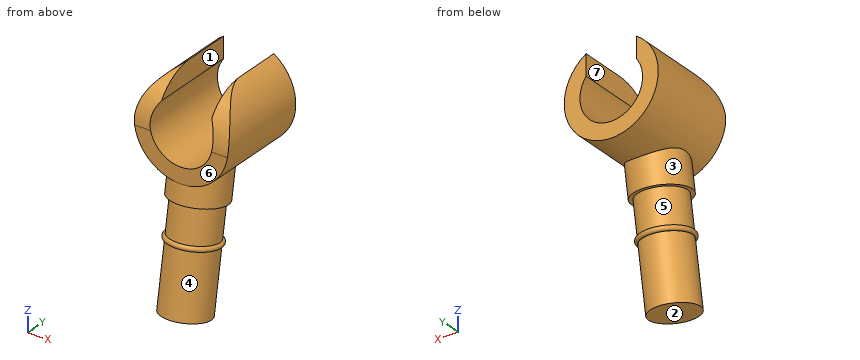
from build123d import *

# Parameters (mm, degrees)
SKETCH2_R                = 2.38125
SKETCH2_R_2              = 1.5875000000000001
BOSS_EXTRUDE1_DEPTH      = 4.7625
SKETCH3_W                = 2.54
SKETCH3_H                = 2.54
CUT_EXTRUDE1_DEPTH       = 6.832847450002443
CUT_EXTRUDE2_DEPTH       = 7.456267061932925
CUT_EXTRUDE2_DEPTH_BACK  = 7.456267061932925
BOSS_EXTRUDE2_REACH      = 13.721
BOSS_EXTRUDE2_END_RADIUS = 2.38125
SKETCH6_R                = 1.1906250000000003
BOSS_EXTRUDE3_REACH      = 19.432
BOSS_EXTRUDE3_END_RADIUS = 2.38125
BOSS_EXTRUDE3_START      = -5.159375
SKETCH7_R                = 1.3881469237206399
SKETCH8_R                = 0.1270000000001564


with BuildPart() as part:
    # Sketch2 → Boss-Extrude1 (new body)
    with BuildSketch(Plane(origin=(0, 0, 0), x_dir=(1, 0, 0), z_dir=(0, 1, 0))):
        with Locations(Location((0, 0, 0), (0, 0, 90))):
            Circle(SKETCH2_R)
        with Locations(Location((0, 0, 0), (0, 0, 90))):
            Circle(SKETCH2_R_2, mode=Mode.SUBTRACT)
    extrude(amount=BOSS_EXTRUDE1_DEPTH)

    # Sketch3 → Cut-Extrude1 (cut, through all)
    with BuildSketch(Plane(origin=(0, 4.7625, 0), x_dir=(1, 0, 0), z_dir=(0, 1, 0))):
        with Locations((0, -2.2225)):
            Rectangle(SKETCH3_W, SKETCH3_H)
    extrude(amount=-CUT_EXTRUDE1_DEPTH, mode=Mode.SUBTRACT)

    # Sketch4 → Cut-Extrude2 (cut, two sides: drawn at the far end of the back side and taken through both)
    with BuildSketch(Plane(origin=(-1.27, 0, 0), x_dir=(0, 0, -1), z_dir=(1, 0, 0)).offset(-CUT_EXTRUDE2_DEPTH_BACK)):
        with BuildLine():
            Line((0.3669383154536387, 0), (-2.014311684546361, 0))
            Line((-2.014311684546361, 0), (-2.0143116845463607, 2.38125))
            ThreePointArc((-2.0143116845463607, 2.38125), (-1.3168597072468262, 0.6974519772995338), (0.3669383154536387, 0))
        make_face()
    extrude(amount=CUT_EXTRUDE2_DEPTH + CUT_EXTRUDE2_DEPTH_BACK, mode=Mode.SUBTRACT)

    # Boss-Extrude2: up to this cylinder (the profile starts outside it)
    boss_extrude2_end = Plane(origin=(0, 0.31226100000000034, 0), z_dir=(0, -1, 0)) * Cylinder(BOSS_EXTRUDE2_END_RADIUS, 33.2045, mode=Mode.PRIVATE)
    # Sketch6 → Boss-Extrude2 (add, up to the surface)
    with BuildSketch(Plane(origin=(0, 0.48483407181496907, -8.634779231627519), x_dir=(-1, 0, 0), z_dir=(0, -0.17364817766693408, -0.9848077530122075)), mode=Mode.PRIVATE) as boss_extrude2_sk1:
        with Locations(Location((4.3e-16, -0.17523538418624157, 0), (0, 0, 90))):
            Circle(SKETCH6_R)
    boss_extrude2_tool1 = extrude(boss_extrude2_sk1.sketch, amount=-BOSS_EXTRUDE2_REACH, mode=Mode.PRIVATE) - boss_extrude2_end
    add(boss_extrude2_tool1.solids().sort_by_distance((0, 0.312261, -8.60435))[0])

    # Boss-Extrude3: up to this cylinder (the profile starts outside it)
    boss_extrude3_end = Plane(origin=(0, 1.208177, 0), z_dir=(0, -1, 0)) * Cylinder(BOSS_EXTRUDE3_END_RADIUS, 44.6265, mode=Mode.PRIVATE)
    # Sketch7 → Boss-Extrude3 (add, up to the surface)
    with BuildSketch(Plane(origin=(0, -1.4620146790809783, -8.291497269485987), x_dir=(-1, 0, 0), z_dir=(0, -0.1736481776669341, -0.9848077530122075)).offset(BOSS_EXTRUDE3_START), mode=Mode.PRIVATE) as boss_extrude3_sk1:
        with Locations(Location((4.3e-16, 1.8016466467900256, 0), (0, 0, 90))):
            Circle(SKETCH7_R)
    boss_extrude3_tool1 = extrude(boss_extrude3_sk1.sketch, amount=-BOSS_EXTRUDE3_REACH, mode=Mode.PRIVATE) - boss_extrude3_end
    add(boss_extrude3_tool1.solids().sort_by_distance((0, 1.208177, -3.523357))[0])

    # Sketch8 → Revolve1 (revolve)
    with BuildSketch(Plane(origin=(0, 0, 0), x_dir=(0, 0, -1), z_dir=(1, 0, 0))):
        with Locations((5.55625, 2.0587154735803463)):
            Circle(SKETCH8_R)
    revolve(axis=Axis((-4.3e-16, 2.2625512819876596, 2.4562964209001934), (0, -0.17364817766693408, -0.9848077530122075)))


solid = part.part
Design review of the part built by this model. Coordinates are the model's own, in mm. Face numbers are marked on the shaded views. A direction names the side the tool comes from. Coordinates: 2 decimals unless noted, no trailing zeros. Loops run counter-clockwise (first coordinate to the right, second up) from the corner with the lowest first, then second, coordinate; pieces in that order, holes last. Notation, with made-up numbers: M -29.5,78 L 7.5,78 A29 ccw 7.5,109 Z; hole C -26,-13 d7. An arc over 180 degrees is marked long. Use one line per item in the form item = value.
(1) Consider section D-D (x = -1.9). Write out the cut boundary in (y, z), and give its area (3 significant figures).
Return value:
outline = M 0,-1.44 L 4.76,-1.44 L 4.76,1.44 L 0.82,1.44 A2.38 ccw 0,-0.37 Z
area = 13.2 mm2
(2) Draft analysis for pull direction Z (two halves, no side actions). For the marked faces 1, 2, 3 and 4, state which applies: pulls with the +Z half, pulls with the -Z half, needs draft (parallel to the pull), parting line crosses it, or undercut.
Return value:
face_1 = needs draft
face_2 = pulls with the -Z half
face_3 = undercut
face_4 = undercut
(3) Consider section C-C (y = 4.4). Write out the cut boundary in (x, z) (1 decimal).
Return value:
outline = M -1.3,1 L -1.3,2 A2.4 ccw long 1.3,2 L 1.3,1 A1.6 cw long Z
(4) Consider section A-A (z = 0). Write out the cut boundary in (x, y).
Return value:
outline = M -2.38,0.03 L -1.59,0.03 L -1.59,4.76 L -2.38,4.76 Z; M 1.59,0.03 L 2.38,0.03 L 2.38,4.76 L 1.59,4.76 Z
(5) For line 1 along Y through (x, z) = (1, -2); line 2 along X through (y, z) = (3.7, 0); line 3 along Z through (x, y) = (1.45, 0.85), list the stretches that pass through material, from the lowest coordinate up. Write a range as from..to.
Return value:
line_1 = 0..4.76
line_2 = -2.38..-1.59, 1.59..2.38
line_3 = -1.89..-0.65, 0.65..1.46
(6) For the marked faces 5, 6 and 7, list the 3-axis set-ups (+Z, -Z, +X, -X, +Y, -Y) from which the entire face can be reached by the end or side of a thin tool; tool diameter is ignored.
Return value:
face_5 = none
face_6 = +Z, +X, -X, -Y
face_7 = +Z, +Y, -Y
(7) Clearance check with flat-ended pins moving along their axes: P1, Ø1.5, axis at y = 2, z = -6.5, coming from the -X side; P2, Ø2, axis at x = 1, z = -1, coming from the -Y side; P3, Ø1.9, axis at x = 0, z = 0, coming from the +Y side; P4, Ø0.8, axis at y = 2, z = 1.5, coming from the -X side. State where each tip first meets the part, or that it passes through.
Return value:
P1 = -1.06
P2 = 0
P3 = through
P4 = -2.11
(8) Consider section B-B (z = -1.25). Write out the cut boundary in (x, y), and give its area (3 significant figures).
Return value:
outline = M -2.03,0 L -0.98,0 L -0.98,4.76 L -2.03,4.76 Z; M 0.98,0 L 2.03,0 L 2.03,4.76 L 0.98,4.76 Z
area = 9.98 mm2
